The model under review builds one solid part; all positions refer to its coordinate system, in mm. Round coordinates to 2 decimals unless told otherwise and drop trailing zeros. Loops run counter-clockwise (first coordinate to the right, second up) from the corner with the lowest first, then second, coordinate; pieces in that order, holes last. Notation, with made-up numbers: M 57.5,-37 L 71.5,-37 A23 ccw 71.5,-29 Z; hole C 68.25,-33.75 d11. An arc over 180 degrees is marked long. Answer in a Markdown table with one row per item. Add a question column.
from build123d import *

# Parameters (mm, degrees)
BOSS_EXTRUDE1_DEPTH = 5
SKETCH2_R           = 13
CUT_EXTRUDE1_DEPTH  = 5


with BuildPart() as part:
    # Sketch1 → Boss-Extrude1 (new body)
    with BuildSketch(Plane(origin=(0, 0, 0), x_dir=(1, 0, 0), z_dir=(0, 1, 0))):
        with BuildLine():
            Line((67.945120995, -67.73797404), (67.945120995, -107.53797404))
            ThreePointArc((67.945120995, -107.53797404), (66.422076258, -111.214929302), (62.745120995, -112.73797404))
            Line((62.745120995, -112.73797404), (-46.431495334, -112.73797404))
            ThreePointArc((-46.431495334, -112.73797404), (-49.244562585, -111.911376907), (-51.163293943, -109.694378902))
            Line((-51.163293943, -109.694378902), (-140.925822463, 87.271513299))
            ThreePointArc((-140.925822463, 87.271513299), (-141.064719238, 91.248996543), (-138.350428716, 94.159716769))
            Line((-138.350428716, 94.159716769), (-97.584163781, 112.73797404))
            Line((-97.584163781, 112.73797404), (-14.302507037, 112.73797404))
            Line((-14.302507037, 112.73797404), (67.945120995, -67.73797404))
        make_face()
    extrude(amount=BOSS_EXTRUDE1_DEPTH)

    # Sketch2 → Cut-Extrude1 (cut)
    with BuildSketch(Plane(origin=(0, 5, 0), x_dir=(1, 0, 0), z_dir=(0, 1, 0))):
        with Locations(Location((-4.347057053, -67.73797404, 0), (0, 0, 270))):
            Circle(SKETCH2_R)
        with Locations(Location((-68.624509665, 73.306022946, 0), (0, 0, 270))):
            Circle(SKETCH2_R)
    extrude(amount=-CUT_EXTRUDE1_DEPTH, mode=Mode.SUBTRACT)


solid = part.part
1. Take a section at D-D, the plane x = 31.5. State the section outline as (y, z) points, and give its area (3 significant figures).
2. To check wall thickness, follow probe 1 along Z at (x, y) = (3, 0.5); probe 2 along X at (y, z) = (4.45, 61.5); probe 3 along Z at (x, y) = (-58.5, 3.7). State the ranges of each line that lie inside material, in increasing order.
3. Take a section at B-B, the plane y = 1.75. State the section outline as (x, z) points.
4. Take a section at A-A, the plane z = -80.5. State the section outline as (x, y) points, and give its area (3 significant figures).
5. For pin 1 Ø3 at (x, y) = (28.5, 4) entering from -Z; pin 2 Ø3 at (y, z) = (1.5, -48) entering from -X; pin 3 Ø2 at (y, z) = (2, -51) entering from -X, all flat-tipped, find the tip position at first contact; note any pin that passes through.
6. Mouldability with a two-part tool opening along X and no side actions: class faces 1 (the flat face through (-57, 2, -112.738)), 2 (the cylindrical face through (-49.209, 2.465, 111.934)), 3 (the cylindrical face through (-59.84, 2.54, -82.89)), 4 (the flat face through (67.945, 2, 87)) as released by +X, released by -X, zero draft, split by the parting line, or undercut.
7. Take a section at C-C, the plane x = -65. State the section outline as (y, z) points.
Check sheet entries:
| question | item | result |
|---|---|---|
| 1 | outline | M 0,-12.23 L 5,-12.23 L 5,112.74 L 0,112.74 Z |
| 1 | area | 625 mm^2 |
| 2 | probe 1 | z = -74.77 to 57.01, 78.46 to 112.74 |
| 2 | probe 2 | x = -73.13 to -15.75, 7.06 to 65.1 |
| 2 | probe 3 | z = -112.74 to -81.46, -65.15 to 93.6 |
| 3 | outline | M -140.93,-87.27 A5.2 ccw -138.35,-94.16 L -97.58,-112.74 L -14.3,-112.74 L 67.95,67.74 L 67.95,107.54 A5.2 ccw 62.75,112.74 L -46.43,112.74 A5.2 ccw -51.16,109.69 Z; hole C -68.62,-73.31 d26; hole C -4.35,67.74 d26 |
| 4 | outline | M -137.84,0 L -79.45,0 L -79.45,5 L -137.84,5 Z; M -57.8,0 L 0.39,0 L 0.39,5 L -57.8,5 Z |
| 4 | area | 583 mm^2 |
| 5 | pin 1 | stops at z = -22.11 |
| 5 | pin 2 | stops at x = -123.71 |
| 5 | pin 3 | stops at x = -124.85 |
| 6 | face 1 | zero draft |
| 6 | face 2 | released by -X |
| 6 | face 3 | undercut |
| 6 | face 4 | released by +X |
| 7 | outline | M 0,-112.74 L 5,-112.74 L 5,-85.79 L 0,-85.79 Z; M 0,-60.82 L 5,-60.82 L 5,79.33 L 0,79.33 Z |
